```python
from build123d import *

# Parameters (mm, degrees)
SKETCH_1_R               = 2.772053215
SKETCH_1_R_2             = 2
SKETCH_1_R_3             = 3.5
EXTRUDE_1_DEPTH          = 1.45
SKETCH_2_R               = 3.5
SKETCH_2_R_2             = 2.35
EXTRUDE_2_DEPTH          = 2.3
SKETCH_3_R               = 2.3
CUT_EXTRUDE_1_DEPTH      = 0.7
SKETCH_4_R               = 1.3
CUT_EXTRUDE_2_DEPTH      = 17.659906963
SKETCH_5_R               = 0.5
CUT_EXTRUDE_3_DEPTH      = 17.8021576
PATTERN_LINEAR_1_COUNT   = 6
PATTERN_LINEAR_1_PITCH   = 2
MIRROR_1_COPY_1_SKETCH_R = 0.5
MIRROR_1_COPY_1_DEPTH    = 17.8021576
MIRROR_1_COPY_2_SKETCH_R = 0.5
MIRROR_1_COPY_2_DEPTH    = 17.8021576
MIRROR_1_COPY_3_SKETCH_R = 0.5
MIRROR_1_COPY_3_DEPTH    = 17.8021576
MIRROR_1_COPY_4_SKETCH_R = 0.5
MIRROR_1_COPY_4_DEPTH    = 17.8021576
MIRROR_1_COPY_5_SKETCH_R = 0.5
MIRROR_1_COPY_5_DEPTH    = 17.8021576


with BuildPart() as part:
    # 草图1 → 凸台-拉伸1 (new body)
    with BuildSketch(Plane.XY):
        with BuildLine():
            Line((0.152869496, 2.767834884), (-1.980633731, 2.885669771))
            ThreePointArc((-1.980633731, 2.885669771), (-3.5, 0), (-1.980633731, -2.885669771))
            Line((-1.980633731, -2.885669771), (0.152869466, -2.767834886))
            ThreePointArc((0.152869466, -2.767834886), (-2.772053215, 1.5e-08), (0.152869496, 2.767834884))
        make_face()
        with BuildLine():
            Line((2.286372673, 2.65), (0.152869496, 2.767834884))
            ThreePointArc((0.152869496, 2.767834884), (2.013459884, 1.90532368), (2.772053215, 0))
            ThreePointArc((2.772053215, 0), (2.013459873, -1.905323691), (0.152869466, -2.767834886))
            Line((0.152869466, -2.767834886), (2.286372673, -2.65))
            ThreePointArc((2.286372673, -2.65), (3.182161557, -1.457342726), (3.5, 0))
            ThreePointArc((3.5, 0), (3.182161557, 1.457342726), (2.286372673, 2.65))
        make_face()
        Circle(SKETCH_1_R)
        with BuildLine():
            ThreePointArc((2.286372673, 2.65), (0.193013304, 3.494673928), (-1.980633731, 2.885669771))
            Line((-1.980633731, 2.885669771), (0.152869496, 2.767834884))
            Line((0.152869496, 2.767834884), (2.286372673, 2.65))
        make_face()
        with BuildLine():
            Line((0.152869466, -2.767834886), (-1.980633731, -2.885669771))
            ThreePointArc((-1.980633731, -2.885669771), (0.193013304, -3.494673928), (2.286372673, -2.65))
            Line((2.286372673, -2.65), (0.152869466, -2.767834886))
        make_face()
        with BuildLine():
            Line((14.11029331, 1.996956531), (2.286372673, 2.65))
            ThreePointArc((2.286372673, 2.65), (3.182161557, 1.457342726), (3.5, 0))
            ThreePointArc((3.5, 0), (3.182161557, -1.457342726), (2.286372673, -2.65))
            Line((2.286372673, -2.65), (14.110293326, -1.99695653))
            ThreePointArc((14.110293326, -1.99695653), (12, -8e-09), (14.11029331, 1.996956531))
        make_face()
        with Locations((14, 0)):
            Circle(SKETCH_1_R_2)
        Circle(SKETCH_1_R_3)
    extrude_1 = extrude(amount=EXTRUDE_1_DEPTH)

    # 草图2 → 凸台-拉伸2 (add)
    with BuildSketch(Plane.XY.offset(1.45)):
        with Locations(Location((0, 0, 0), (0, 0, 310.787038193))):
            Circle(SKETCH_2_R)
        Circle(SKETCH_2_R_2, mode=Mode.SUBTRACT)
    extrude(amount=EXTRUDE_2_DEPTH)

    # 草图3 → 切除-拉伸1 (cut)
    with BuildSketch(Plane(origin=(0, 0, 0), x_dir=(-1, 0, 0), z_dir=(0, 0, -1))):
        Circle(SKETCH_3_R)
    cut_extrude_1 = extrude(amount=-CUT_EXTRUDE_1_DEPTH, mode=Mode.SUBTRACT)

    # 草图4 → 切除-拉伸2 (cut, through all)
    with BuildSketch(Plane(origin=(0, 0, 0.7), x_dir=(-1, 0, 0), z_dir=(0, 0, -1))):
        Circle(SKETCH_4_R)
    cut_extrude_2 = extrude(amount=-CUT_EXTRUDE_2_DEPTH, mode=Mode.SUBTRACT)

    # 草图5 → 切除-拉伸3 (cut, through all)
    with BuildSketch(Plane(origin=(0, 0, 0), x_dir=(-1, 0, 0), z_dir=(0, 0, -1))):
        with Locations((-14.4, 0)):
            Circle(SKETCH_5_R)
    cut_extrude_3 = extrude(amount=-CUT_EXTRUDE_3_DEPTH, mode=Mode.SUBTRACT)

    # 阵列(线性)1: 切除-拉伸3 ×6
    with Locations(*[(-i * PATTERN_LINEAR_1_PITCH, 0, 0) for i in range(1, PATTERN_LINEAR_1_COUNT)]):
        add(cut_extrude_3, mode=Mode.SUBTRACT)

    # 镜向1: 凸台-拉伸1, 切除-拉伸1, 切除-拉伸2, 切除-拉伸3 across plane
    add(extrude_1.mirror(Plane(origin=(0, 0, 0), x_dir=(0, 0, 1), z_dir=(1, 0, 0))))
    add(cut_extrude_1.mirror(Plane(origin=(0, 0, 0), x_dir=(0, 0, 1), z_dir=(1, 0, 0))), mode=Mode.SUBTRACT)
    add(cut_extrude_2.mirror(Plane(origin=(0, 0, 0), x_dir=(0, 0, 1), z_dir=(1, 0, 0))), mode=Mode.SUBTRACT)
    add(cut_extrude_3.mirror(Plane(origin=(0, 0, 0), x_dir=(0, 0, 1), z_dir=(1, 0, 0))), mode=Mode.SUBTRACT)

    # 镜向1 copy 1 sketch → 镜向1 copy 1 (cut, through all)
    with BuildSketch(Plane(origin=(2, 0, 0), x_dir=(1, 0, 0), z_dir=(0, 0, -1))):
        with Locations((-14.4, 0)):
            Circle(MIRROR_1_COPY_1_SKETCH_R)
    extrude(amount=-MIRROR_1_COPY_1_DEPTH, mode=Mode.SUBTRACT)

    # 镜向1 copy 2 sketch → 镜向1 copy 2 (cut, through all)
    with BuildSketch(Plane(origin=(4, 0, 0), x_dir=(1, 0, 0), z_dir=(0, 0, -1))):
        with Locations((-14.4, 0)):
            Circle(MIRROR_1_COPY_2_SKETCH_R)
    extrude(amount=-MIRROR_1_COPY_2_DEPTH, mode=Mode.SUBTRACT)

    # 镜向1 copy 3 sketch → 镜向1 copy 3 (cut, through all)
    with BuildSketch(Plane(origin=(6, 0, 0), x_dir=(1, 0, 0), z_dir=(0, 0, -1))):
        with Locations((-14.4, 0)):
            Circle(MIRROR_1_COPY_3_SKETCH_R)
    extrude(amount=-MIRROR_1_COPY_3_DEPTH, mode=Mode.SUBTRACT)

    # 镜向1 copy 4 sketch → 镜向1 copy 4 (cut, through all)
    with BuildSketch(Plane(origin=(8, 0, 0), x_dir=(1, 0, 0), z_dir=(0, 0, -1))):
        with Locations((-14.4, 0)):
            Circle(MIRROR_1_COPY_4_SKETCH_R)
    extrude(amount=-MIRROR_1_COPY_4_DEPTH, mode=Mode.SUBTRACT)

    # 镜向1 copy 5 sketch → 镜向1 copy 5 (cut, through all)
    with BuildSketch(Plane(origin=(10, 0, 0), x_dir=(1, 0, 0), z_dir=(0, 0, -1))):
        with Locations((-14.4, 0)):
            Circle(MIRROR_1_COPY_5_SKETCH_R)
    extrude(amount=-MIRROR_1_COPY_5_DEPTH, mode=Mode.SUBTRACT)


solid = part.part
```
Build history of the part. All positions in model axes, mm. A direction names the side the tool comes from. Coordinates: 2 decimals unless noted, no trailing zeros. Write each loop counter-clockwise with the first axis right and the second up, starting at its lowest first coordinate (ties: lowest second). Pieces come first, ordered by that corner, then holes.
1. Band-saw the part on A-A, the plane x = -12.4. Give the cut face in (y, z).
Answer block:
outline: (-2.09, 0) - (-0.5, 0) - (-0.5, 1.45) - (-2.09, 1.45) - close; (0.5, 0) - (2.09, 0) - (2.09, 1.45) - (0.5, 1.45) - close
2. Drop flat-ended pins along their axis: pin 1 (1.5 mm diameter, centred on x = 12.5, y = 0, fed in from +Z); pin 2 (1.5 mm diameter, centred on x = 5, z = 1, fed in from -Y); pin 3 (1.5 mm diameter, centred on y = -2.5, z = 0.5, fed in from -X); pin 4 (2 mm diameter, centred on x = -10.5, z = 2.5, fed in from -Y). Give the stop position or say it passes through.
Answer block:
pin 1: stops at z = 1.45
pin 2: stops at y = -2.54
pin 3: stops at x = -14.97
pin 4: passes through
3. Band-saw the part on B-B, the plane z = 1. Give the number of separate pieces and of enclosed holes in the cut face, and give its area (3 significant figures).
Answer block:
separate pieces: 1
enclosed holes: 13
area: 136 mm2
4. Band-saw the part on D-D, the plane z = 3.05. Give the cut face in (x, y), and give its area (3 significant figures).
Answer block:
outline: circle Ø7 at (0, 0); hole circle Ø4.7 at (0, 0)
area: 21.1 mm2
5. Band-saw the part on C-C, the plane y = 1. Give the cut face in (x, z).
Answer block:
outline: (-15.73, 0) - (-2.07, 0) - (-2.07, 0.7) - (-0.83, 0.7) - (-0.83, 1.45) - (-2.13, 1.45) - (-2.13, 3.75) - (-3.35, 3.75) - (-3.35, 1.45) - (-15.73, 1.45) - close; (0.83, 0.7) - (2.07, 0.7) - (2.07, 0) - (15.73, 0) - (15.73, 1.45) - (3.35, 1.45) - (3.35, 3.75) - (2.13, 3.75) - (2.13, 1.45) - (0.83, 1.45) - close
6. 3-axis set-ups, long thin cutter, end or side, ignore diameter. For faces 5 (the cylindrical face through (14.9, 0, 0.7)), 6 (the cylindrical face through (-0.509, -2.294, 2.584)): which of +Z, -Z, +X, -X, +Y, -Y reach the whole face in a straight line?
Answer block:
face 5: +Z, -Z
face 6: +Z
7. Drill centre lines: probe 1 along Y at (x, z) = (0, 2.8); probe 2 along Z at (x, y) = (9.5, 0); probe 3 along X at (y, z) = (-1, 1.7). Where is each one in solid material? Low to high.
Answer block:
probe 1: y = -3.5 to -2.35, 2.35 to 3.5
probe 2: z = 0 to 1.45
probe 3: x = -3.35 to -2.13, 2.13 to 3.35
8. Pull direction X, two halves, no side cores. Call faces 1 (the flat face through (8.116, -2.328, 0.715)), 2 (the cylindrical face through (10.9, 0, 0.7)), 3 (the flat face through (2, 2, 3.75)), 4 (the flat face through (-8.116, -2.328, 0.715)): released by +X, released by -X, zero draft, split by the parting line, or undercut.
Answer block:
face 1: released by +X
face 2: undercut
face 3: zero draft
face 4: released by -X
